from build123d import *

# Parameters (mm, degrees)
F1_DEPTH = 25.4
F2_R     = 6.35
F3_DEPTH = 25.4
F4_R     = 6.35
F5_DEPTH = 25.4


with BuildPart() as f1:
    # F0 (on Front) → F1 (new body)
    with BuildSketch(Plane.XZ):
        Polygon((0, 12.7), (0, 0), (76.2, 0), (76.2, 12.7), (50.8, 12.7), (50.8, 44.45), (25.4, 44.45), (25.4, 12.7), align=None)
    extrude(amount=F1_DEPTH)

    # F2 (on face) → F3 (cut)
    with BuildSketch(Plane.YZ.offset(50.8)):
        with BuildLine():
            ThreePointArc((-25.4, 31.75), (-21.680256, 40.730256), (-12.7, 44.45))
            Line((-12.7, 44.45), (-25.4, 44.45))
            Line((-25.4, 44.45), (-25.4, 31.75))
        make_face()
        with BuildLine():
            ThreePointArc((-12.7, 44.45), (-3.719744, 40.730256), (0, 31.75))
            Line((0, 31.75), (0, 44.45))
            Line((0, 44.45), (-12.7, 44.45))
        make_face()
        with Locations((-12.7, 31.75)):
            Circle(F2_R)
    extrude(amount=-F3_DEPTH, mode=Mode.SUBTRACT)

    # F4 (on face) → F5 (cut)
    with BuildSketch(Plane.XY.offset(12.7)):
        with Locations((63.499989, -12.7)):
            Circle(F4_R)
        with Locations((12.7, -12.7)):
            Circle(F4_R)
        with BuildLine():
            ThreePointArc((63.5, 1.1e-05), (76.2, -12.7), (63.5, -25.400011))
            Line((63.5, -25.400011), (94.457269, -25.400011))
            Line((94.457269, -25.400011), (94.457269, 0))
            Line((94.457269, 0), (63.5, 1.1e-05))
        make_face()
        with BuildLine():
            ThreePointArc((12.7, -25.4), (0.016976, -12.7), (12.7, 0))
            Line((12.7, 0), (0, 0))
            Line((0, 0), (0, -25.4))
            Line((0, -25.4), (12.7, -25.4))
        make_face()
    extrude(amount=-F5_DEPTH, mode=Mode.SUBTRACT)


solid = f1.part
Geometry check sheet. Reference: the model listing, model coordinates, mm. A direction names the side the tool comes from. Round coordinates to 2 decimals unless told otherwise and drop trailing zeros. Write each loop counter-clockwise with the first axis right and the second up, starting at its lowest first coordinate (ties: lowest second). Pieces come first, ordered by that corner, then holes. Notation, with made-up numbers: (1.5, 35) -> (23.5, 35) arc R20 ccw to (23.5, 69) -> close; hole circle Ø2 at (77.5, 58.25). An arc over 180 degrees is marked (long way). One line per item, written item: value. Start each with the question number.
(1) Cross-section at A-A, the plane y = -16. Record the cut outline in (x, z).
(2) Draft check along Y on faces 1 (the flat face through (38, -25.4, 13)), 2 (the cylindrical face through (57.156, -12.421, 6.439)), 3 (the cylindrical face through (7.66, -16.56, 6.44)), 4 (the flat face through (38, 0, 13)). Enter one of: +Y half, -Y half, draft (parallel to the pull), parting line (faces both ways), or undercut.
(3) Go/stop test with flat-tipped pins: pin 1 Ø5 at (y, z) = (-22.5, 36) entering from +X; pin 2 Ø6 at (y, z) = (-18.5, 21) entering from -X; pin 3 Ø12.5 at (x, y) = (10, -16) entering from +Z. Record where each tip stops, or that it passes through.
(4) Access from +Z, -Z, +X, -X, +Y, -Y to the whole of each face (thin tool, end or side, straight path). Record for faces 5 (the flat face through (25.4, -13, 25)), 6 (the flat face through (55, -13, 12.7)), 7 (the flat face through (38, -13, 0)).
(5) Cross-section at C-C, the plane y = -21.5. Record the cut outline in (x, z), and give its area (3 significant figures).
(6) Cross-section at D-D, the plane z = 22.5. Record the cut outline in (x, y), and give its area (3 significant figures).
(7) Scan lines: line 1 (X direction, y = -16, z = 11); line 2 (Y direction, x = 12.7, z = 7.75); line 3 (Z direction, x = 36, y = -12.7). Record each from-to range of solid material in increasing order. Write a range as [from, to].
(8) Cross-section at B-B, the plane x = 30. Record the cut outline in (y, z), and give its area (3 significant figures).
Answer:
1. outline: (0.45, 0) -> (7.27, 0) -> (7.27, 12.7) -> (0.45, 12.7) -> close; (18.13, 0) -> (58.07, 0) -> (58.07, 12.7) -> (50.8, 12.7) -> (50.8, 26.32) -> (25.4, 26.32) -> (25.4, 12.7) -> (18.13, 12.7) -> close; (25.4, 37.18) -> (50.8, 37.18) -> (50.8, 44.01) -> (25.4, 44.01) -> close; (68.93, 0) -> (75.76, 0) -> (75.76, 12.7) -> (68.93, 12.7) -> close
2. face 1: -Y half
2. face 2: undercut
2. face 3: undercut
2. face 4: +Y half
3. pin 1: x = 50.8
3. pin 2: x = 25.4
3. pin 3: z = 12.7
4. face 5: +Z, -X, +Y, -Y
4. face 6: +Z, +X, +Y, -Y
4. face 7: -Z, +X, -X, +Y, -Y
5. outline: (3.56, 0) -> (72.66, 0) -> (72.66, 12.7) -> (50.8, 12.7) -> (50.8, 40.91) -> (25.4, 40.91) -> (25.4, 12.7) -> (3.56, 12.7) -> close
5. area: 1,590 mm²
6. outline: (25.4, -25.4) -> (50.8, -25.4) -> (50.8, 0) -> (25.4, 0) -> close
6. area: 645 mm²
7. line 1: [0.45, 7.27], [18.13, 58.07], [68.93, 75.76]
7. line 2: [-25.4, -19.05], [-6.35, 0]
7. line 3: [0, 25.4], [38.1, 44.45]
8. outline: (-25.4, 0) -> (0, 0) -> (0, 31.75) arc R12.7 ccw to (-25.4, 31.75) -> close; hole circle Ø12.7 at (-12.7, 31.75)
8. area: 933 mm²
